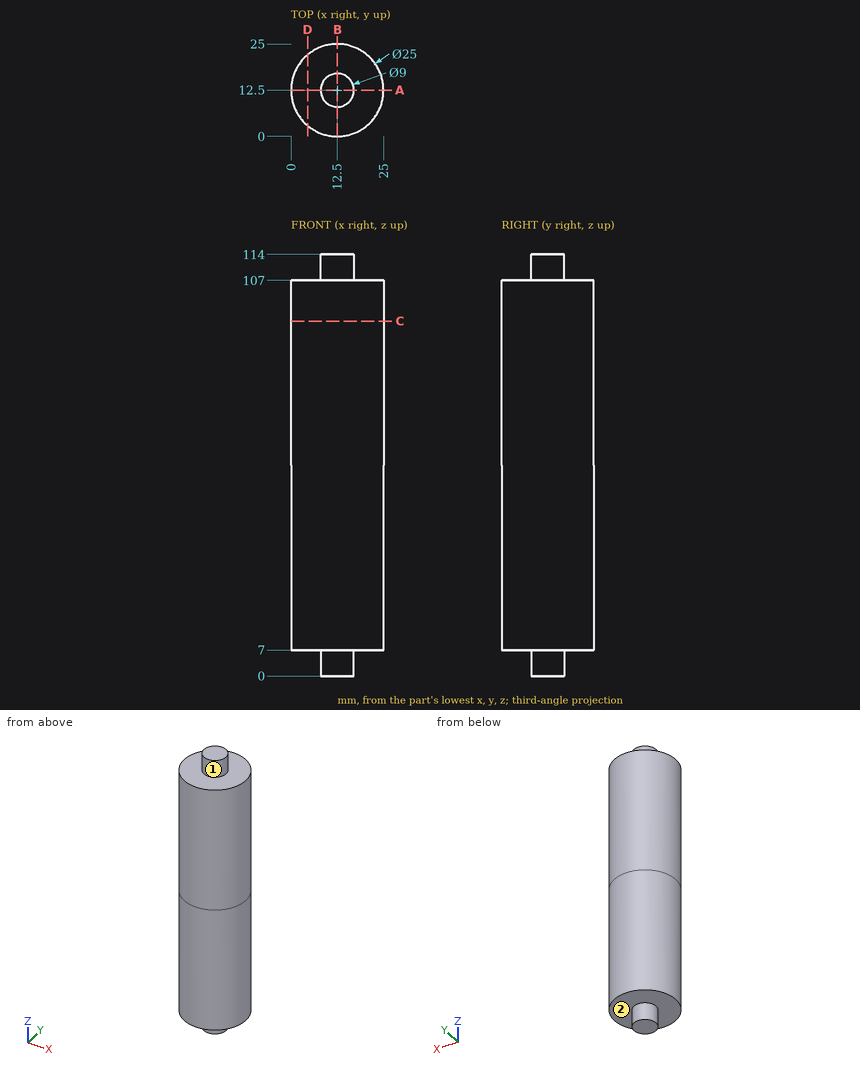
Here's the drawing with two shaded views (mm, measured from the low corner). I have some questions. A direction names the side the tool comes from. Coordinates: 2 decimals unless noted, no trailing zeros. Write each loop counter-clockwise with the first axis right and the second up, starting at its lowest first coordinate (ties: lowest second). Pieces come first, ordered by that corner, then holes.
Item 1: Will these pins go through, and if not, where does the flat tip stop? pin 1 (1 mm diameter, centred on x = 14, y = 22, fed in from +Z); pin 2 (6 mm diameter, centred on y = 16, z = 89.5, fed in from -X); pin 3 (10 mm diameter, centred on x = 3.5, z = 83.5, fed in from -Y).
Item 2: If I drill on line 1 (Z direction, x = 1, y = 7.75); line 2 (Y direction, x = 12, z = 64); line 3 (X direction, y = 13.5, z = 108), over which ranges is the centre line in solid material (lowest first)?
Item 3: I want a section at A-A on y = 12.5. Write out the boundary of the cut face in (x, z).
Item 4: I want a section at D-D on x = 4.5. Write out the boundary of the cut face in (y, z).
Item 5: I want a section at C-C on z = 96. Write out the boundary of the cut face in (x, y).
Item 6: On a 3-axis mill with a long thin cutter (end or side, diameter ignored), from which of +Z, -Z, +X, -X, +Y, -Y can I reach the whole of each face in a straight line? I mean the marked faces 1 and 2. Say none if no direction works.
Findings below:
1. pin 1: stops at z = 107
1. pin 2: stops at x = 0.01
1. pin 3: stops at y = 0.66
2. line 1: z = 7 to 107
2. line 2: y = 0.01 to 24.99
2. line 3: x = 8.11 to 16.89
3. outline: (0, 7) - (8, 7) - (8, 0) - (17, 0) - (17, 7) - (25, 7) - (25, 107) - (17, 107) - (17, 114) - (8, 114) - (8, 107) - (0, 107) - close
4. outline: (2.9, 7) - (22.1, 7) - (22.1, 107) - (2.9, 107) - close
5. outline: circle Ø25 at (12.5, 12.5)
6. face 1: +Z
6. face 2: -Z
